Geometry check sheet. Reference: drawing and pictorial views, mm from the part's lowest x, y, z. A direction names the side the tool comes from. Coordinates: 2 decimals unless noted, no trailing zeros. Write each loop counter-clockwise with the first axis right and the second up, starting at its lowest first coordinate (ties: lowest second). Pieces come first, ordered by that corner, then holes. Notation, with made-up numbers: (65, 3.25) - (75, 3.25) arc R11 cw to (75, 11.25) - close; hole circle Ø10 at (14.5, -28.75). An arc over 180 degrees is marked (long way). Answer as a JSON object with one key per item and string values. Group by question number.
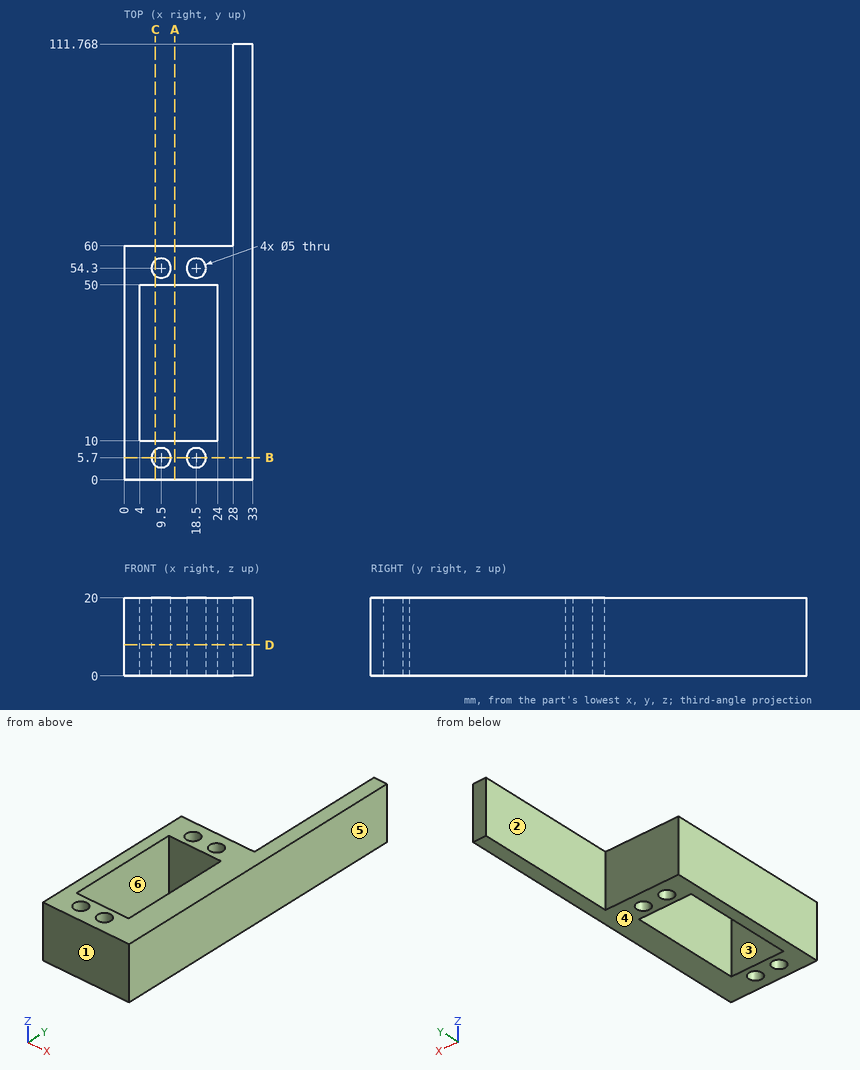
(1) Set-up check for the marked faces 1, 2 and 3: record each of +Z, -Z, +X, -X, +Y, -Y from which the full face is reachable in a straight line by a thin tool's end or side.
(2) Section check D-D (z = 8). Record the cut outline in (x, y), and give its area (3 significant figures).
(3) Material ranges on L1, parallel to Y at x = 18.5, z = 5.75; L2, parallel to X at y = 30, z = 16.75; L3, parallel to Y at x = 14, z = 3, recorded low to high. Write a range as [from, to].
(4) Section check A-A (x = 13). Record the cut outline in (y, z), and give its area (3 significant figures).
(5) Gauge pin test, flat ends, axial feed: pin 1 (6.5 mm diameter, centred on x = 9.5, y = 5.7, fed in from -Z); pin 2 (6 mm diameter, centred on x = 11.5, z = 11.5, fed in from +Y); pin 3 (10 mm diameter, centred on y = 90, z = 5, fed in from -X). Record the tip position at first contact, or that the pin passes through.
(6) Draft check along X on the marked faces 4, 5 and 6. Enter one of: +X half, -X half, draft (parallel to the pull), parting line (faces both ways), or undercut.
(7) Section check C-C (x = 8). Record the cut outline in (y, z), and give its area (3 significant figures).
(8) Section check B-B (y = 5.7). Record the cut outline in (x, z).
Conclusion:
{
 "1": {"face 1": "+Z, -Z, +X, -X, -Y", "face 2": "+Z, -Z, -X, +Y", "face 3": "+Z, -Z"},
 "2": {"outline": "(0, 0) - (33, 0) - (33, 111.77) - (28, 111.77) - (28, 60) - (0, 60) - close; hole (4, 10) - (24, 10) - (24, 50) - (4, 50) - close; hole circle Ø5 at (9.5, 5.7); hole circle Ø5 at (9.5, 54.3); hole circle Ø5 at (18.5, 5.7); hole circle Ø5 at (18.5, 54.3)", "area": "1,360 mm^2"},
 "3": {"L1": "y = [0, 3.2], [8.2, 10], [50, 51.8], [56.8, 60]", "L2": "x = [0, 4], [24, 33]", "L3": "y = [0, 10], [50, 60]"},
 "4": {"outline": "(0, 0) - (10, 0) - (10, 20) - (0, 20) - close; (50, 0) - (60, 0) - (60, 20) - (50, 20) - close", "area": "400 mm^2"},
 "5": {"pin 1": "stops at z = 0", "pin 2": "stops at y = 60", "pin 3": "stops at x = 28"},
 "6": {"face 4": "draft", "face 5": "+X half", "face 6": "undercut"},
 "7": {"outline": "(0, 0) - (3.7, 0) - (3.7, 20) - (0, 20) - close; (7.7, 0) - (10, 0) - (10, 20) - (7.7, 20) - close; (50, 0) - (52.3, 0) - (52.3, 20) - (50, 20) - close; (56.3, 0) - (60, 0) - (60, 20) - (56.3, 20) - close", "area": "240 mm^2"},
 "8": {"outline": "(0, 0) - (7, 0) - (7, 20) - (0, 20) - close; (12, 0) - (16, 0) - (16, 20) - (12, 20) - close; (21, 0) - (33, 0) - (33, 20) - (21, 20) - close"}
}
